from build123d import *

# Parameters (mm, degrees)
BOSS_EXTRUDE1_DEPTH      = 457.2
BOSS_EXTRUDE1_DEPTH_BACK = 457.2
SKETCH6_W                = 114.3
SKETCH6_H                = 63.5
SIDE_CUT_DEPTH           = 466.069768959
TRIANGLE_CUT_DEPTH       = 466.069768959
SKETCH8_R                = 6.35
CUT_EXTRUDE4_DEPTH       = 466.069768959


with BuildPart() as part:
    # Sketch4 → Boss-Extrude1 (new, two sides: drawn at the far end of the back side and taken through both)
    with BuildSketch(Plane.XY.offset(-BOSS_EXTRUDE1_DEPTH_BACK)):
        with BuildLine():
            Line((38.1, -34.29), (38.1, 34.29))
            ThreePointArc((38.1, 34.29), (36.984076836, 36.984076836), (34.29, 38.1))
            Line((34.29, 38.1), (-34.29, 38.1))
            ThreePointArc((-34.29, 38.1), (-36.984076836, 36.984076836), (-38.1, 34.29))
            Line((-38.1, 34.29), (-38.1, -34.29))
            ThreePointArc((-38.1, -34.29), (-36.984076836, -36.984076836), (-34.29, -38.1))
            Line((-34.29, -38.1), (34.29, -38.1))
            ThreePointArc((34.29, -38.1), (36.984076836, -36.984076836), (38.1, -34.29))
        make_face()
        with BuildLine():
            Line((31.75, 28.575), (31.75, -28.575))
            ThreePointArc((31.75, -28.575), (30.82006403, -30.82006403), (28.575, -31.75))
            Line((28.575, -31.75), (-28.575, -31.75))
            ThreePointArc((-28.575, -31.75), (-30.82006403, -30.82006403), (-31.75, -28.575))
            Line((-31.75, -28.575), (-31.75, 28.575))
            ThreePointArc((-31.75, 28.575), (-30.82006403, 30.82006403), (-28.575, 31.75))
            Line((-28.575, 31.75), (28.575, 31.75))
            ThreePointArc((28.575, 31.75), (30.82006403, 30.82006403), (31.75, 28.575))
        make_face(mode=Mode.SUBTRACT)
    extrude(amount=BOSS_EXTRUDE1_DEPTH + BOSS_EXTRUDE1_DEPTH_BACK)

    # Sketch6 → side cut (cut, through all)
    with BuildSketch(Plane.ZY.offset(38.1)):
        with Locations((-400.05, 0)):
            Rectangle(SKETCH6_W, SKETCH6_H)
    extrude(amount=-SIDE_CUT_DEPTH, mode=Mode.SUBTRACT)

    # Sketch7 → triangle cut (cut, through all)
    with BuildSketch(Plane.XZ.offset(38.1)):
        Polygon((-38.1, -342.9), (-38.1, -457.2), (-12.7, -457.2), align=None)
        Polygon((12.7, -457.2), (38.1, -342.9), (38.1, -457.2), align=None)
    extrude(amount=-TRIANGLE_CUT_DEPTH, mode=Mode.SUBTRACT)

    # Sketch8 → Cut-Extrude4 (cut, through all)
    with BuildSketch(Plane(origin=(0, 38.1, 0), x_dir=(1, 0, 0), z_dir=(0, 1, 0))):
        with Locations(Location((0, 441.325, 0), (0, 0, 270))):
            Circle(SKETCH8_R)
    extrude(amount=-CUT_EXTRUDE4_DEPTH, mode=Mode.SUBTRACT)


solid = part.part
Could you check a few things on this model? Use its own coordinates, in mm. A direction names the side the tool comes from. Coordinates: 2 decimals unless noted, no trailing zeros. Order: outer loops, then holes, each group sorted by start corner. A loop starts at its lowest first (then second) coordinate and runs counter-clockwise, first axis right, second up. Notation, with made-up numbers: (38, 17) -> (97, 17) arc R28 cw to (97, 42) -> close; hole circle Ø10 at (-31, 25.5). An arc over 180 degrees is marked (long way). One line per question, with ' | ' between items.
Q1. I'm going to push a flat-ended pin straight in: P1, Ø3, axis at x = 34.5, y = -5, coming from the -Z side. Where does the tip first touch, or does it pass through?
Return value:
P1: z = -342.9
Q2. Imagine slicing it at A-A on z = 300.5. Please give me the cut outline in (x, y) (3 decimals).
Return value:
outline: (-38.1, -34.29) arc R3.81 ccw to (-34.29, -38.1) -> (34.29, -38.1) arc R3.81 ccw to (38.1, -34.29) -> (38.1, 34.29) arc R3.81 ccw to (34.29, 38.1) -> (-34.29, 38.1) arc R3.81 ccw to (-38.1, 34.29) -> close; hole (-31.75, -28.575) arc R3.175 ccw to (-28.575, -31.75) -> (28.575, -31.75) arc R3.175 ccw to (31.75, -28.575) -> (31.75, 28.575) arc R3.175 ccw to (28.575, 31.75) -> (-28.575, 31.75) arc R3.175 ccw to (-31.75, 28.575) -> close
Q3. Thinking about a two-plate mould opening in X: for faces 3 (the face through (-31.75, 0, 52)), 4 (the face through (25.222, 34.881, -400.85)), 5 (the face through (-38.1, 0, 52)), 6 (the face through (0, 38.1, -6)), which applies, pulls with the +X half, pulls with the -X half, needs draft (parallel to the pull), parting line crosses it, or undercut?
Return value:
face 3: undercut | face 4: pulls with the +X half | face 5: pulls with the -X half | face 6: needs draft
Q4. On a 3-axis mill with a long thin cutter (end or side, diameter ignored), from which of +Z, -Z, +X, -X, +Y, -Y can I reach the whole of each face in a straight line? I mean faces 1 (the face through (0, -38.1, -6)), 2 (the face through (31.75, 0, 52)). Say none if no direction works.
Return value:
face 1: +Z, -Z, +X, -X, -Y | face 2: +Z, -Z
Q5. If I drill on L1, parallel to Y at x = 29.5, z = 228; L2, parallel to Y at x = 14, z = 237, over which ranges is the centre line in solid material (lowest first)?
Return value:
L1: -38.1 to -31.61, 31.61 to 38.1 | L2: -38.1 to -31.75, 31.75 to 38.1
Q6. Imagine slicing it at B-B on y = -4.5. Please give me the cut outline in (x, z), and give its area (3 significant figures).
Return value:
outline: (-38.1, -342.9) -> (-31.75, -342.9) -> (-31.75, 457.2) -> (-38.1, 457.2) -> close; (31.75, -342.9) -> (38.1, -342.9) -> (38.1, 457.2) -> (31.75, 457.2) -> close | area: 10,200 mm²
